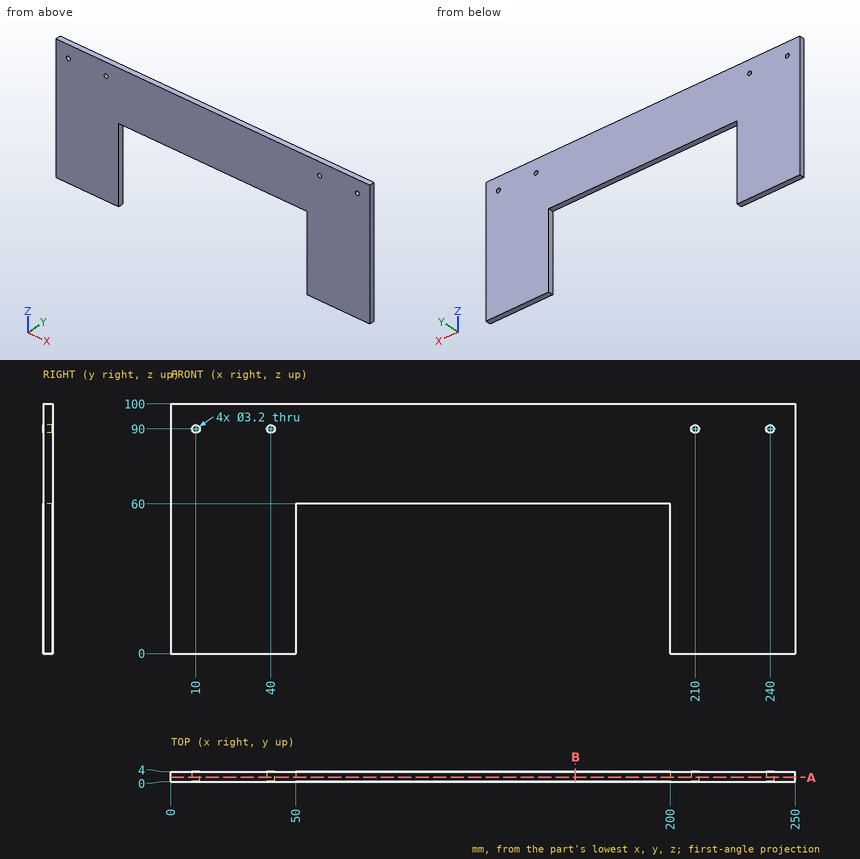
Could you check a few things on this drawing? It's one solid part, dimensions in mm from its lowest x, y, z. Round coordinates to 2 decimals unless told otherwise and drop trailing zeros. Write each loop counter-clockwise with the first axis right and the second up, starting at its lowest first coordinate (ties: lowest second). Pieces come first, ordered by that corner, then holes. Notation, with made-up numbers: (68.25, -37) -> (120.25, -37) arc R27 cw to (120.25, 0) -> close; hole circle Ø4 at (14.5, 41.5). An arc over 180 degrees is marked (long way). One line per item, written item: value.
1) I'm going to push flat-ended pins straight in: pin 1 Ø3 at (x, z) = (40, 90) entering from -Y; pin 2 Ø2 at (x, y) = (101, 3) entering from -Z. Where does each tip first touch, or does it pass through?
Filled sheet:
pin 1: passes through
pin 2: stops at z = 60
2) Suppose I cut it at A-A on y = 1.65. List the corners of the cut face in (x, z) for me.
Filled sheet:
outline: (0, 0) -> (50, 0) -> (50, 60) -> (200, 60) -> (200, 0) -> (250, 0) -> (250, 100) -> (0, 100) -> close; hole circle Ø3.2 at (10, 90); hole circle Ø3.2 at (40, 90); hole circle Ø3.2 at (210, 90); hole circle Ø3.2 at (240, 90)
3) If I drill on line 1 (X direction, y = 2.7, z = 90); line 2 (X direction, y = 2.75, z = 53); line 3 (Z direction, x = 10, y = 1.4), over which ranges is the centre line in solid material (lowest first)? Write a range as [from, to].
Filled sheet:
line 1: x = [0, 8.4], [11.6, 38.4], [41.6, 208.4], [211.6, 238.4], [241.6, 250]
line 2: x = [0, 50], [200, 250]
line 3: z = [0, 88.4], [91.6, 100]
4) Suppose I cut it at B-B on x = 162. List the corners of the cut face in (y, z) for me, plus the area to 3 significant figures.
Filled sheet:
outline: (0, 60) -> (4, 60) -> (4, 100) -> (0, 100) -> close
area: 160 mm2
